Check sheet for the drawn part. Datum: minimum x, y, z corner. Units: mm. Coordinates: 2 decimals unless noted, no trailing zeros. Order: outer loops, then holes, each group sorted by start corner. A loop starts at its lowest first (then second) coordinate and runs counter-clockwise, first axis right, second up. Notation, with made-up numbers: (0, 61) - (14, 61) arc R20 ccw to (14, 80) - close; hole circle Ø8 at (-6.75, -34). An arc over 180 degrees is marked (long way). Answer as CSV lines item,"result". Start each with the question number.
1. Material ranges on L1, parallel to Z at x = 30, y = 6; L2, parallel to X at y = 43.5, z = 2.75; L3, parallel to X at y = 69, z = 6, recorded low to high. Write a range as [from, to].
2. Section check B-B (z = 3). Record the cut outline in (x, y) (1 decimal).
3. Section check A-A (y = 42.5). Record the cut outline in (x, z).
4. Go/stop test with flat-tipped pins: pin 1 (4 mm diameter, centred on x = 41.5, z = 3, fed in from -Y); pin 2 (2 mm diameter, centred on y = 40, z = 2, fed in from +X); pin 3 (1.2 mm diameter, centred on y = 19.5, z = 6, fed in from -X); pin 4 (5 mm diameter, centred on x = 49, y = 39, fed in from -Z). Record where each tip stops, or that it passes through.
5. Section check C-C (x = 56). Record the cut outline in (y, z).
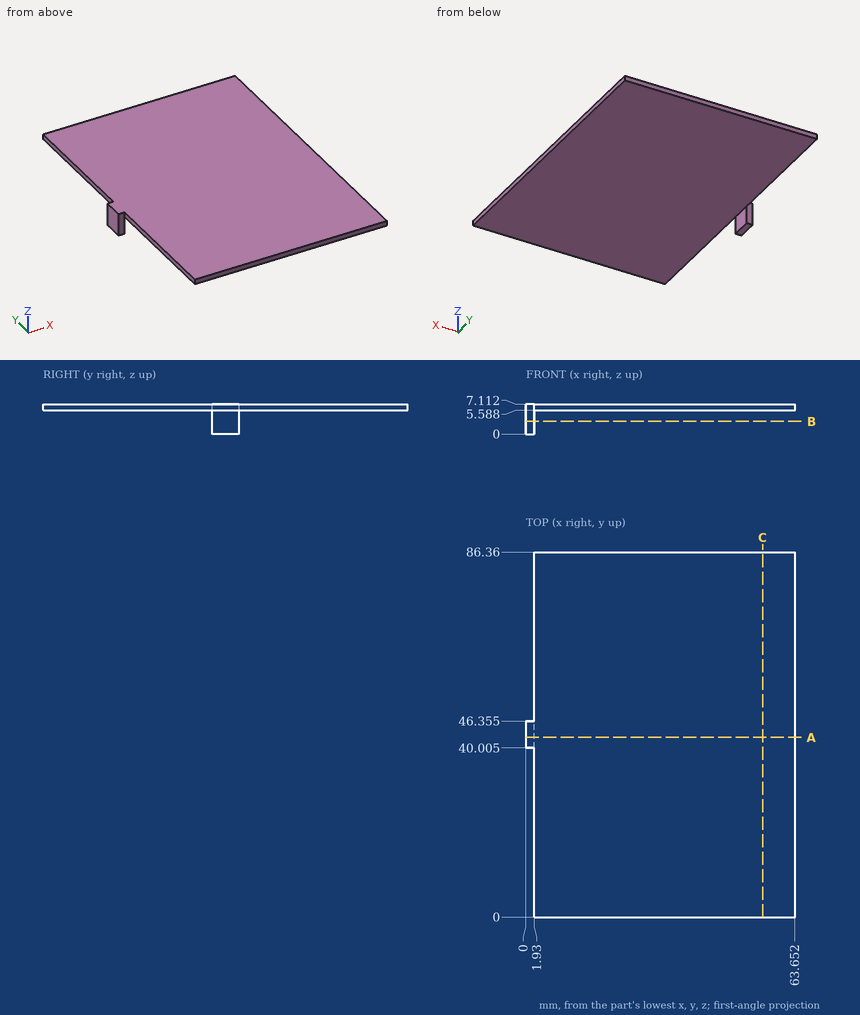
Evaluation:
1,L1,"z = [5.59, 7.11]"
1,L2,"x = [0, 1.93]"
1,L3,"x = [1.93, 63.65]"
2,outline,"(0, 40) - (1.9, 40) - (1.9, 46.4) - (0, 46.4) - close"
3,outline,"(0, 0) - (1.93, 0) - (1.93, 5.59) - (63.65, 5.59) - (63.65, 7.11) - (0, 7.11) - close"
4,pin 1,"passes through"
4,pin 2,"stops at x = 1.93"
4,pin 3,"stops at x = 1.93"
4,pin 4,"stops at z = 5.59"
5,outline,"(0, 5.59) - (86.36, 5.59) - (86.36, 7.11) - (0, 7.11) - close"
